from build123d import *

# Parameters (mm, degrees)
BOSS_EXTRUDE1_DEPTH = 22
SKETCH2_R           = 4
BOSS_EXTRUDE2_DEPTH = 17
BOSS_EXTRUDE3_DEPTH = 10
SKETCH4_R           = 9.25
BOSS_EXTRUDE4_DEPTH = 18
SKETCH5_R           = 10
BOSS_EXTRUDE5_DEPTH = 9
BOSS_EXTRUDE6_DEPTH = 10
SKETCH7_R           = 6
BOSS_EXTRUDE7_DEPTH = 6
SKETCH8_R           = 6
BOSS_EXTRUDE8_DEPTH = 6


with BuildPart() as part:
    # Sketch1 → Boss-Extrude1 (new body)
    with BuildSketch(Plane(origin=(0, 0, 0), x_dir=(1, 0, 0), z_dir=(0, 1, 0))):
        Polygon((0, 0), (80, 0), (80, 34.5), (0, 34.5), (0, 65), (-29, 65), (-29, 6), (0, 6), align=None)
    extrude(amount=BOSS_EXTRUDE1_DEPTH)

    # Sketch2 → Boss-Extrude2 (add)
    with BuildSketch(Plane.XY):
        with Locations((30.5, 11)):
            Circle(SKETCH2_R)
        with Locations((66.5, 11)):
            Circle(SKETCH2_R)
    extrude(amount=BOSS_EXTRUDE2_DEPTH)

    # Sketch3 → Boss-Extrude3 (add)
    with BuildSketch(Plane(origin=(0, 0, -34.5), x_dir=(-1, 0, 0), z_dir=(0, 0, -1))):
        Polygon((-50.834192463, 11), (-54.875644347, 18), (-62.958548116, 18), (-67, 11), (-62.958548116, 4), (-54.875644347, 4), align=None)
        Polygon((-29.668384925, 11), (-33.70983681, 18), (-41.792740578, 18), (-45.834192463, 11), (-41.792740578, 4), (-33.70983681, 4), align=None)
    extrude(amount=BOSS_EXTRUDE3_DEPTH)

    # Sketch4 → Boss-Extrude4 (add)
    with BuildSketch(Plane(origin=(0, 0, 0), x_dir=(0, 0, -1), z_dir=(1, 0, 0))):
        with Locations((56.75, 11)):
            Circle(SKETCH4_R)
    extrude(amount=BOSS_EXTRUDE4_DEPTH)

    # Sketch5 → Boss-Extrude5 (add)
    with BuildSketch(Plane.ZY.offset(29)):
        with Locations((-17.7, 11)):
            Circle(SKETCH5_R)
    extrude(amount=BOSS_EXTRUDE5_DEPTH)

    # Sketch6 → Boss-Extrude6 (add)
    with BuildSketch(Plane.XY):
        Polygon((56.582903769, 11), (52.541451884, 18), (44.458548116, 18), (40.417096231, 11), (44.458548116, 4), (52.541451884, 4), align=None)
    extrude(amount=BOSS_EXTRUDE6_DEPTH)

    # Sketch7 → Boss-Extrude7 (add)
    with BuildSketch(Plane.XY.offset(10)):
        with Locations((48.5, 11)):
            Circle(SKETCH7_R)
    extrude(amount=BOSS_EXTRUDE7_DEPTH)

    # Sketch8 → Boss-Extrude8 (add)
    with BuildSketch(Plane(origin=(0, 0, -44.5), x_dir=(-1, 0, 0), z_dir=(0, 0, -1))):
        with Locations((-58.917096231, 11)):
            Circle(SKETCH8_R)
        with Locations((-37.751288694, 11)):
            Circle(SKETCH8_R)
    extrude(amount=BOSS_EXTRUDE8_DEPTH)


solid = part.part
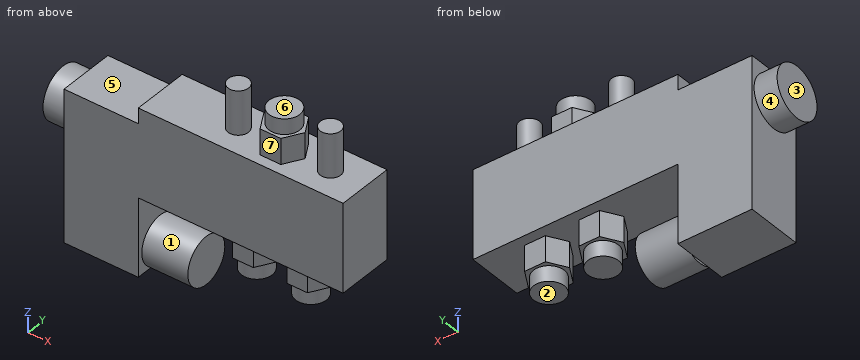
Verification items for the finished model (mm, model axes). Face numbers are marked on the shaded views. A direction names the side the tool comes from. Give positions to 0.01 mm unless a question says otherwise; leave off trailing zeros. Write each loop counter-clockwise with the first axis right and the second up, starting at its lowest first coordinate (ties: lowest second). Pieces come first, ordered by that corner, then holes. Notation, with made-up numbers: M -3,15 L 45,15 A28 cw 45,34 Z; hole C 46,25.25 d3. An arc over 180 degrees is marked long. Put each result on its own line as item: value. Start each with the question number.
1. Section check B-B (x = -24). Record the cut outline in (y, z), and give its area (3 significant figures).
2. Set-up check for the marked faces 5, 6 and 7: record each of +Z, -Z, +X, -X, +Y, -Y from which the full face is reachable in a straight line by a thin tool's end or side.
3. Section check C-C (x = 22). Record the cut outline in (y, z).
4. Section check A-A (z = -56.75). Record the cut outline in (x, y), and give its area (3 significant figures).
5. Scan lines: line 1 along X through (y, z) = (8.75, -46); line 2 along X through (y, z) = (17.75, -26.5); line 3 along X through (y, z) = (21.25, -38.5). Record each from-to range of solid material in increasing order. Write a range as [from, to].
6. Draft check along Z on the marked faces 1, 2, 3 and 4. Enter one of: +Z half, -Z half, draft (parallel to the pull), parting line (faces both ways), or undercut.
7. Go/stop test with flat-tipped pins: pin 1 Ø5 at (y, z) = (18.5, -37) entering from -X; pin 2 Ø11 at (x, y) = (-16, 15.5) entering from -Z; pin 3 Ø9 at (x, z) = (57, -40) entering from +Y. Record where each tip stops, or that it passes through.
Answer list:
1. outline: M 0,-65 L 22,-65 L 22,-6 L 0,-6 Z
1. area: 1,300 mm2
2. face 5: +Z, -X, +Y, -Y
2. face 6: +Z, +Y, -Y
2. face 7: +Z, +X, -X, -Y
3. outline: M 0,-34.5 L 22,-34.5 L 22,0 L 0,0 Z
4. outline: M -29,0 L 0,0 L 0,1.75 L 18,1.75 L 18,20.25 L 0,20.25 L 0,22 L -29,22 Z
4. area: 971 mm2
5. line 1: [-29, 0], [32.19, 43.31], [53.35, 64.48]
5. line 2: [-29, 80]
5. line 3: [-29, 0]
6. face 1: undercut
6. face 2: -Z half
6. face 3: draft
6. face 4: parting line
7. pin 1: x = -29
7. pin 2: z = -65
7. pin 3: y = 18
